from build123d import *

# Parameters (mm, degrees)
SM_BASE_FLANGE_1_DEPTH = 104
SKETCH_7_R             = 2.75
CUT_EXTRUDE_3_DEPTH    = 3
SKETCH_8_R             = 25.78
CUT_EXTRUDE_4_DEPTH    = 3
SKETCH_9_R             = 4.4
CUT_EXTRUDE_5_DEPTH    = 3


# Sheet-metal steps are written as plain solids
with BuildPart() as part:
    # Sketch 1 → 基体-法兰1 (new body)
    with BuildSketch(Plane.XY):
        with BuildLine():
            Line((-70, -35), (-70, -4))
            ThreePointArc((-70, -4), (-68.828427125, -1.171572875), (-66, 0))
            Line((-66, 0), (66, 0))
            ThreePointArc((66, 0), (68.828427125, -1.171572875), (70, -4))
            Line((70, -4), (70, -35))
            Line((70, -35), (67, -35))
            Line((67, -35), (67, -4))
            ThreePointArc((67, -4), (66.707106781, -3.292893219), (66, -3))
            Line((66, -3), (-66, -3))
            ThreePointArc((-66, -3), (-66.707106781, -3.292893219), (-67, -4))
            Line((-67, -4), (-67, -35))
            Line((-67, -35), (-70, -35))
        make_face()
    extrude(amount=SM_BASE_FLANGE_1_DEPTH)

    # 草图7 → 切除-拉伸3 (cut)
    with BuildSketch(Plane.ZY.offset(70)):
        with Locations(Location((38, -29, 0), (0, 0, 270))):
            Circle(SKETCH_7_R)
        with Locations(Location((38, -11, 0), (0, 0, 270))):
            Circle(SKETCH_7_R)
        with Locations(Location((6, -11, 0), (0, 0, 270))):
            Circle(SKETCH_7_R)
        with Locations(Location((6, -29, 0), (0, 0, 270))):
            Circle(SKETCH_7_R)
    cut_extrude_3 = extrude(amount=-CUT_EXTRUDE_3_DEPTH, mode=Mode.SUBTRACT)

    # 镜向2: 切除-拉伸3 across plane
    add(cut_extrude_3.mirror(Plane(origin=(0, 0, 0), x_dir=(0, 0, 1), z_dir=(1, 0, 0))), mode=Mode.SUBTRACT)

    # 草图8 → 切除-拉伸4 (cut)
    with BuildSketch(Plane(origin=(0, 0, 0), x_dir=(1, 0, 0), z_dir=(0, 1, 0))):
        with Locations(Location((0, -52, 0), (0, 0, 270))):
            Circle(SKETCH_8_R)
    extrude(amount=-CUT_EXTRUDE_4_DEPTH, mode=Mode.SUBTRACT)

    # 草图9 → 切除-拉伸5 (cut)
    with BuildSketch(Plane(origin=(0, 0, 0), x_dir=(1, 0, 0), z_dir=(0, 1, 0))):
        with Locations(Location((-40, -12, 0), (0, 0, 270))):
            Circle(SKETCH_9_R)
        with Locations(Location((40, -12, 0), (0, 0, 270))):
            Circle(SKETCH_9_R)
        with Locations(Location((-40, -92, 0), (0, 0, 270))):
            Circle(SKETCH_9_R)
        with Locations(Location((40, -92, 0), (0, 0, 270))):
            Circle(SKETCH_9_R)
    extrude(amount=-CUT_EXTRUDE_5_DEPTH, mode=Mode.SUBTRACT)


solid = part.part
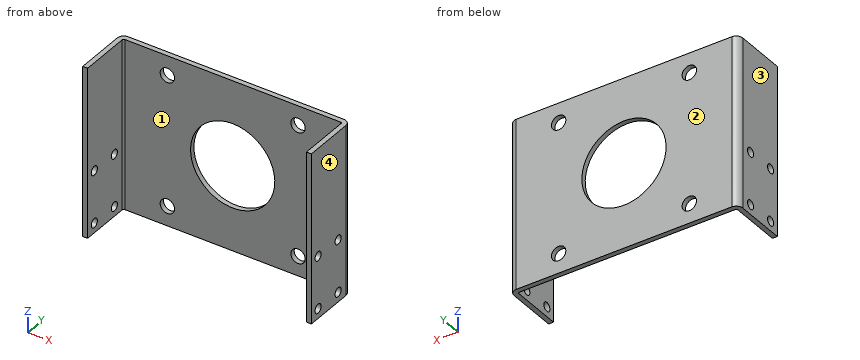
Read the model definition and answer for the solid it produces. Units are mm, in the model's axes. Face numbers are marked on the shaded views. Round coordinates to 2 decimals unless told otherwise and drop trailing zeros. Order: outer loops, then holes, each group sorted by start corner. A loop starts at its lowest first (then second) coordinate and runs counter-clockwise, first axis right, second up.
1) The part is cut by section D-D on x = -21. Write down the section's boundary in (y, z).
2) The part is cut by section A-A on x = -40. Write down the section's boundary in (y, z).
3) The mould has two halves that part along X. Classify the marked faces 1, 2, 3 and 4: released by +X, released by -X, zero draft, split by the parting line, or undercut.
4) The part is cut by section B-B on y = -29. Write down the section's boundary in (x, z).
5) Straight lines are drawn through the part: L1, parallel to Z at x = 67.9, y = -29; L2, parallel to X at y = -5, z = 32.5; L3, parallel to X at y = -2, z = 89.5. For each, find the intervals that lie inside material, in ascending order.
6) A flat-ended cylindrical pin translates along its axis: pin 1 (4.5 mm diameter, centred on y = -29, z = 6, fed in from +X). Find the tip coordinate at first contact, or state that the pin passes through.
7) The part is cut by section C-C on z = 6. Write down the section's boundary in (x, y).
Resolved:
1. outline: (-3, 0) - (0, 0) - (0, 37.05) - (-3, 37.05) - close; (-3, 66.95) - (0, 66.95) - (0, 104) - (-3, 104) - close
2. outline: (-3, 0) - (0, 0) - (0, 7.6) - (-3, 7.6) - close; (-3, 16.4) - (0, 16.4) - (0, 87.6) - (-3, 87.6) - close; (-3, 96.4) - (0, 96.4) - (0, 104) - (-3, 104) - close
3. face 1: undercut
3. face 2: zero draft
3. face 3: released by -X
3. face 4: released by +X
4. outline: (-70, 0) - (-67, 0) - (-67, 3.25) - (-70, 3.25) - close; (-70, 8.75) - (-67, 8.75) - (-67, 35.25) - (-70, 35.25) - close; (-70, 40.75) - (-67, 40.75) - (-67, 104) - (-70, 104) - close; (67, 0) - (70, 0) - (70, 3.25) - (67, 3.25) - close; (67, 8.75) - (70, 8.75) - (70, 35.25) - (67, 35.25) - close; (67, 40.75) - (70, 40.75) - (70, 104) - (67, 104) - close
5. L1: z = 0 to 3.25, 8.75 to 35.25, 40.75 to 104
5. L2: x = -70 to -67, 67 to 70
5. L3: x = -69.46 to -43.62, -36.38 to 36.38, 43.62 to 69.46
6. pin 1: passes through
7. outline: (-70, -35) - (-67, -35) - (-67, -31.75) - (-70, -31.75) - close; (-70, -26.25) - (-67, -26.25) - (-67, -13.75) - (-70, -13.75) - close; (-70, -8.25) - (-67, -8.25) - (-67, -4) arc R1 cw to (-66, -3) - (66, -3) arc R1 cw to (67, -4) - (67, -8.25) - (70, -8.25) - (70, -4) arc R4 ccw to (66, 0) - (-66, 0) arc R4 ccw to (-70, -4) - close; (67, -35) - (70, -35) - (70, -31.75) - (67, -31.75) - close; (67, -26.25) - (70, -26.25) - (70, -13.75) - (67, -13.75) - close
